Autodesk Inventor part; units mm, degrees
ref_plane "Work Plane1" through (29, 0, 0) normal (0, -1, 0) x (1, 0, 0)
ref_plane "YZ Plane" through (0, 0, 0) normal (1, 0, 0) x (0, 1, 0)
ref_plane "XZ Plane" through (0, 0, 0) normal (0, 1, 0) x (-1, 0, 0)
sketch "Sketch1" plane through (0, 0, 0) normal (0, 0, 1) x (1, 0, 0)
  line L0 (-1.016, 0) -> (31.75, 0)
  line L1 (31.75, 0) -> (31.75, 2.0828)
  line L2 (31.75, 2.0828) -> (9.652, 2.0828)
  line L3 (9.652, 2.0828) -> (7.6677, 2.0828)
  line L4 (7.6677, 2.0828) -> (0, 2.0828)
  line L5 (0, 2.0828) -> (0, 3.429)
  line L6 (0, 3.429) -> (-4.1656, 3.429)
  line L7 (-4.1656, 3.429) -> (-4.1656, 2.0677)
  line L8 (-4.1656, 2.0677) -> (-2.2098, 2.0677)
  line L9 (-2.2098, 2.0677) -> (-1.016, 0)
  line L10 (-11.3487, 0) -> (38.9331, 0)
  line L11 (0, -0.6858) -> (0, 4.1148)
  line L12 (9.652, 2.0828) -> (0, 2.0828) construction
  dimension "d1" = 22.098
  dimension "d2" = 1.9844
  dimension "d3" = 4.1656
  dimension "d4" = 1.9558
  dimension "d5" = 60
  dimension "d6" = 4.1656
  dimension "d7" = 4.1656
  dimension "d8" = 4.1354
  dimension "d9" = 6.858
  dimension "d26" = 31.75
revolve "Body" add sketch "Sketch1" angle 360 about axis through (-1.016, 0, 0) along (1, 0, 0)
sketch "Sketch2" plane through (-4.1656, 0, 0) normal (-1, 0, 0) x (0, 0, 1)
  circle A0 centre (0, 0) radius 2.0677
  line L0 (0, -4.8006) -> (0, 4.8006)
  line L1 (-4.8006, 0) -> (4.8006, 0)
  line L2 (2.0677, 0) -> (1.0339, -1.7907)
  line L3 (1.0339, -1.7907) -> (-1.0339, -1.7907)
  line L4 (-1.0339, -1.7907) -> (-2.0677, 0)
  line L5 (-2.0677, 0) -> (-1.0339, 1.7907)
  line L6 (-1.0339, 1.7907) -> (1.0339, 1.7907)
  line L7 (1.0339, 1.7907) -> (2.0677, 0)
extrude "Slot" add sketch "Sketch2" against normal up to next contours L7 A0 | A0 L2 | L6 L0 A0 | A0 L0 L3 | L0 L6 A0 | A0 L3 L0 | L4 A0 | A0 L5
fillet "Fillet1" radius 0.3556 1 edges at (-4.1656, -3.429, 0)
thread "Thread"
chamfer "Chamfer1" distance 0.4724 distance2 0.4724 1 edges at (31.75, -2.0828, 0) measured on face at (31.75, 0.2462, 0.6492)
ref_plane "Work Plane1" through (29, 0, 0) normal (0, -1, 0) x (1, 0, 0)
fillet "Fillet2" radius 0.1524 1 edges at (0, -2.0828, 0)
equation "\"d1\" = GEL"
equation "\"d3\" = KOH"
equation "\"d4\" = INTI"
equation "\"d6\" = GD"
equation "\"d7\" = BDM"
equation "\"d8\" = 1.1547 * SW"
equation "\"d9\" = KOD"
equation "\"d26\" = NLG"
equation "\"d30\" = R"
equation "\"d17\" = RR"
equation "\"d13\" = GEL"
equation "\"d15\" = -0.5 * SPD + 0.5 * GD"
equation "\"d16\" = GUL"
equation "\"GD\" = 4.1656"
equation "\"NLG\" = 31.75"
equation "\"GEL\" = 22.098"
equation "\"KOD\" = 6.858"
equation "\"KOH\" = 4.1656"
equation "\"INTI\" = 1.9558"
equation "\"GAL\" = 1.98425"
equation "\"GUL\" = 0.47244"
equation "\"BDM\" = 4.1656"
equation "\"SW\" = 3.5814"
equation "\"RR\" = 0.3556"
equation "\"SPD\" = 3.22072"
equation "\"R\" = 0.1524"
equation "\"PHH\" = 0.127"
equation "\"GD1\" = SPD"
equation "\"THREADDIA\" = 4.1656"
equation "\"FAWI\" = 45deg"
equation "\"KOH1\" = 3.7592"
equation "\"NND\" = 4.1656"
equation "\"TOA\" = 30deg"
equation "\"E0\" = 1.155 * SW"
properties part number "ANSI B18.3 - No. 8 - 32 UNC - 1 1/4 HS HCS" material "Steel, Mild"
The listing builds one solid part. Answer for the finished solid, in the listing's coordinates (mm). A direction names the side the tool comes from. Round coordinates to 2 decimals unless told otherwise and drop trailing zeros. Loops run counter-clockwise (first coordinate to the right, second up) from the corner with the lowest first, then second, coordinate; pieces in that order, holes last. Notation, with made-up numbers: M -40,10.5 L -36,10.5 A18 cw -36,34.5 Z; hole C 63.25,55.5 d2. An arc over 180 degrees is marked long. Return JSON: item names as keys, results as strings.
Q1. The mould has two halves that part along Z. Classify faces 3 (the face through (-3.12, 0.88, -1.56)), 4 (the face through (15.497, 1.987, -0.626)), 5 (the face through (-4.166, -2, 0)): released by +Z, released by -Z, zero draft, split by the parting line, or undercut.
Results list:
{"face 3": "undercut", "face 4": "split by the parting line", "face 5": "zero draft"}
Q2. Which of the six approach directions +Z, -Z, +X, -X, +Y, -Y give full straight-line access (tool end or side, diameter ignored) to faces 1 (the face through (-3, 1.791, 0)), 2 (the face through (-1.93, -0.74, 3.35))?
Results list:
{"face 1": "-X", "face 2": "+X, -X"}
Q3. Find section A-A, the plane x = 15. Determine the outline of the cut face in (y, z), plus the area to 3 significant figures.
Results list:
{"outline": "C 0,0 d4.17", "area": "13.6 mm2"}
Q4. Each of these flat-tipped pins is pushed along its axis until it touches: pin 1 Ø4 at (x, y) = (15.5, -2) entering from +Z; pin 2 Ø1 at (x, z) = (10.5, -0.5) entering from -Y; pin 3 Ø0.6 at (x, z) = (-3, 0.5) entering from +Y. Where does it stop, or does it pass through?
Results list:
{"pin 1": "stops at z = 2.08", "pin 2": "stops at y = -2.08", "pin 3": "stops at y = 3.42"}
Q5. Find the intervals of material crossed by line 1 along Y through (x, z) = (19, 0.25); line 2 along X through (y, z) = (-2.25, -2), in increasing order. Write a range as from..to.
Results list:
{"line 1": "y = -2.07..2.07", "line 2": "x = -4.17..0"}
